from build123d import *

# Parameters (mm, degrees)
SKETCH1_W           = 20
SKETCH1_H           = 8
SKETCH1_R           = 2.75
BOSS_EXTRUDE1_DEPTH = 20
SKETCH2_W           = 14
SKETCH2_H           = 8
CUT_EXTRUDE1_DEPTH  = 16
SKETCH3_R           = 2.75
CUT_EXTRUDE2_DEPTH  = 26.922962794


with BuildPart() as part:
    # Sketch1 → Boss-Extrude1 (new body)
    with BuildSketch(Plane.XY):
        Rectangle(SKETCH1_W, SKETCH1_H)
        with Locations((6, 0)):
            Circle(SKETCH1_R, mode=Mode.SUBTRACT)
    extrude(amount=BOSS_EXTRUDE1_DEPTH)

    # Sketch2 → Cut-Extrude1 (cut)
    with BuildSketch(Plane(origin=(10, 0, 0), x_dir=(0, 0, -1), z_dir=(1, 0, 0))):
        with Locations((-10, 0)):
            Rectangle(SKETCH2_W, SKETCH2_H)
    extrude(amount=-CUT_EXTRUDE1_DEPTH, mode=Mode.SUBTRACT)

    # Sketch3 → Cut-Extrude2 (cut, through all)
    with BuildSketch(Plane(origin=(-6, 0, 0), x_dir=(0, 0, -1), z_dir=(1, 0, 0))):
        with Locations((-10, 0)):
            Circle(SKETCH3_R)
    extrude(amount=-CUT_EXTRUDE2_DEPTH, mode=Mode.SUBTRACT)


solid = part.part
The model under review builds one solid part; all positions refer to its coordinate system, in mm. A direction names the side the tool comes from. Give positions to 0.01 mm unless a question says otherwise; leave off trailing zeros. Write each loop counter-clockwise with the first axis right and the second up, starting at its lowest first coordinate (ties: lowest second). Pieces come first, ordered by that corner, then holes.
1. Add section D-D, the plane x = -2.5. Write out the cut boundary in (y, z), plus the area to 3 significant figures.
2. Add section A-A, the plane z = 10. Write out the cut boundary in (x, y).
3. Add section B-B, the plane x = 6. Write out the cut boundary in (y, z), plus the area to 3 significant figures.
4. Draft analysis for pull direction Y (two halves, no side actions). For faces 3 (the flat face through (-7, -4, 10)), 4 (the flat face through (-10, -1.8, 7.6)), 5 (the cylindrical face through (8.54, -1.05, 1.48)), state which applies: +Y half, -Y half, draft (parallel to the pull), parting line (faces both ways), or undercut.
5. Add section C-C, the plane y = 0. Write out the cut boundary in (x, z).
6. Wall thickness on L1, parallel to Z at x = -2, y = 0.25; L2, parallel to Y at x = -7.85, z = 10; L3, parallel to X at y = 0, z = 19.3: over which ranges is each line inside the solid? List them lowest first.
7. Tool access review of faces 1 (the flat face through (0, 0, 3)), 2 (the flat face through (0, 0, 0)): name each direction out of +Z, -Z, +X, -X, +Y, -Y from which nothing blocks a thin tool from reaching the whole face with its end or side.
8. For P1, Ø4, axis at y = 1, z = 12.5, coming from the +X side; P2, Ø2, axis at x = 5, y = -0.5, coming from the +Z side, all flat-tipped, find the tip position at first contact; note any pin that passes through.
Worked answers:
1. outline: (-4, 0) - (4, 0) - (4, 3) - (-4, 3) - close; (-4, 17) - (4, 17) - (4, 20) - (-4, 20) - close
1. area: 48.0 mm2
2. outline: (-10, -4) - (-6, -4) - (-6, -2.75) - (-10, -2.75) - close; (-10, 2.75) - (-6, 2.75) - (-6, 4) - (-10, 4) - close
3. outline: (-4, 0) - (-2.75, 0) - (-2.75, 3) - (-4, 3) - close; (-4, 17) - (-2.75, 17) - (-2.75, 20) - (-4, 20) - close; (2.75, 0) - (4, 0) - (4, 3) - (2.75, 3) - close; (2.75, 17) - (4, 17) - (4, 20) - (2.75, 20) - close
3. area: 15.0 mm2
4. face 3: -Y half
4. face 4: draft
4. face 5: undercut
5. outline: (-10, 0) - (3.25, 0) - (3.25, 3) - (-6, 3) - (-6, 7.25) - (-10, 7.25) - close; (-10, 12.75) - (-6, 12.75) - (-6, 17) - (3.25, 17) - (3.25, 20) - (-10, 20) - close; (8.75, 0) - (10, 0) - (10, 3) - (8.75, 3) - close; (8.75, 17) - (10, 17) - (10, 20) - (8.75, 20) - close
6. L1: z = 0 to 3, 17 to 20
6. L2: y = -4 to -2.75, 2.75 to 4
6. L3: x = -10 to 3.25, 8.75 to 10
7. face 1: +X, +Y, -Y
7. face 2: -Z, +X, -X, +Y, -Y
8. P1: stops at x = -6
8. P2: passes through
